from build123d import *

# Parameters (mm, degrees)
SKETCH_1_R          = 16
SKETCH_1_R_2        = 8
EXTRUDE_1_DEPTH     = 14
SKETCH_2_R          = 20
SKETCH_2_R_2        = 10
CUT_EXTRUDE_1_DEPTH = 12
EXTRUDE_START       = -5
SKETCH_4_R          = 9.5
SKETCH_4_R_2        = 7.5
EXTRUDE_2_DEPTH     = 4
EXTRUDE_START_2     = 17
SKETCH_6_R          = 16
SKETCH_6_R_2        = 14
EXTRUDE_3_DEPTH     = 17
EXTRUDE_START_3     = 3
SKETCH_7_R          = 21
SKETCH_7_R_2        = 14
EXTRUDE_4_DEPTH     = 3
SKETCH_8_R          = 1.5
CUT_EXTRUDE_4_DEPTH = 10
SKETCH_11_W         = 15
SKETCH_11_H         = 15
CUT_EXTRUDE_5_DEPTH = 11


with BuildPart() as part:
    # 草图1 → 凸台-拉伸1 (new body)
    with BuildSketch(Plane(origin=(0, 0, 0), x_dir=(1, 0, 0), z_dir=(0, 1, 0))):
        with Locations(Location((0, 0, 0), (0, 0, 270))):
            Circle(SKETCH_1_R)
        with Locations(Location((0, 0, 0), (0, 0, 270))):
            Circle(SKETCH_1_R_2, mode=Mode.SUBTRACT)
    extrude(amount=EXTRUDE_1_DEPTH)

    # 草图2 → 切除-拉伸1 (cut)
    with BuildSketch(Plane(origin=(0, 14, 0), x_dir=(1, 0, 0), z_dir=(0, 1, 0))):
        Circle(SKETCH_2_R)
        with Locations(Location((0, 0, 0), (0, 0, 270))):
            Circle(SKETCH_2_R_2, mode=Mode.SUBTRACT)
    extrude(amount=-CUT_EXTRUDE_1_DEPTH, mode=Mode.SUBTRACT)

    # 草图4 → 凸台-拉伸2 (add)
    with BuildSketch(Plane.XZ.offset(EXTRUDE_START)):
        Circle(SKETCH_4_R)
        with Locations(Location((0, 0, 0), (0, 0, 270))):
            Circle(SKETCH_4_R_2, mode=Mode.SUBTRACT)
    extrude(amount=-EXTRUDE_2_DEPTH)

    # 草图6 → 凸台-拉伸3 (add)
    with BuildSketch(Plane.XZ.offset(EXTRUDE_START_2)):
        with Locations(Location((0, 0, 0), (0, 0, 270))):
            Circle(SKETCH_6_R)
        with Locations(Location((0, 0, 0), (0, 0, 270))):
            Circle(SKETCH_6_R_2, mode=Mode.SUBTRACT)
    extrude(amount=-EXTRUDE_3_DEPTH)

    # 草图7 → 凸台-拉伸4 (add)
    with BuildSketch(Plane.XZ.offset(17).offset(EXTRUDE_START_3)):
        with Locations(Location((0, 0, 0), (0, 0, 270))):
            Circle(SKETCH_7_R)
        with Locations(Location((0, 0, 0), (0, 0, 270))):
            Circle(SKETCH_7_R_2, mode=Mode.SUBTRACT)
    extrude(amount=-EXTRUDE_4_DEPTH)

    # 草图8 → 切除-拉伸4 (cut)
    with BuildSketch(Plane(origin=(0, -17, 0), x_dir=(1, 0, 0), z_dir=(0, 1, 0))):
        with Locations(Location((18.5, 0, 0), (0, 0, 270))):
            Circle(SKETCH_8_R)
        with Locations(Location((-9.25, -16.02146997, 0), (0, 0, 270))):
            Circle(SKETCH_8_R)
        with Locations(Location((-9.25, 16.02146997, 0), (0, 0, 270))):
            Circle(SKETCH_8_R)
    extrude(amount=-CUT_EXTRUDE_4_DEPTH, mode=Mode.SUBTRACT)

    # 草图11 → 切除-拉伸5 (cut, symmetric)
    with BuildSketch(Plane.XY):
        with Locations((-8.5, -8.5)):
            Rectangle(SKETCH_11_W, SKETCH_11_H)
    cut_extrude_5 = extrude(amount=CUT_EXTRUDE_5_DEPTH, both=True, mode=Mode.SUBTRACT)

    # 镜向1: 切除-拉伸5 across plane
    add(cut_extrude_5.mirror(Plane(origin=(0, 0, 0), x_dir=(0, 0, 1), z_dir=(1, 0, 0))), mode=Mode.SUBTRACT)


solid = part.part
Input: part model. Units: mm. Frame: model coordinates. A direction names the side the tool comes from. Coordinates: 2 decimals unless noted, no trailing zeros. Write each loop counter-clockwise with the first axis right and the second up, starting at its lowest first coordinate (ties: lowest second). Pieces come first, ordered by that corner, then holes. Notation, with made-up numbers: M 55,85 L 109,85 A20 cw 109,106 Z; hole C -39,-4.5 d11. An arc over 180 degrees is marked long. Answer as a JSON object with one key per item and string values. Group by question number.
(1) Set-up query: faces 1 (the face through (-9.76, 8.08, -2.17)), 2 (the face through (-10, -8, 11)), 3 (the face through (6.31, -18.52, -20.03)), 4 (the face through (-6, 0, 6)). Return all of +Z, -Z, +X, -X, +Y, -Y with unobstructed straight access to the full face (end or side cutting, diameter ignored); none if empty.
(2) Ray query, line 1 along X through (y, z) = (-18, 0); line 2 along Y through (x, z) = (13.5, -4.5); line 3 along X through (y, z) = (6.8, 0). Return the intervals inside material, ascending. Write a range as [from, to].
(3) Mould query, pull axis Y, two halves, no side actions, for faces 5 (the face through (10, -8, 11)), 6 (the face through (0.33, 6.972, 7.493)), 7 (the face through (-15.5, -17, -4.6)). Classes: pulls with the +Y half, pulls with the -Y half, needs draft (parallel to the pull), parting line crosses it, or undercut.
(4) Section B-B on x = -9.25. Give the number of separate pieces and of enclosed holes in the cut face, plus the area to 3 significant figures.
(5) Contact query for flat-ended pins moving along their axis: P1, Ø0.9, axis at x = 10.5, y = -10.5, coming from the +Z side; P2, Ø8, axis at x = -4.5, y = 0, coming from the -Z side; P3, Ø8, axis at x = 3, z = -2.5, coming from the -Y side; P4, Ø9.5, axis at x = 0, z = 0, coming from the -Y side. Output: stop coordinate, or through.
(6) Section A-A on x = 0. Output: boundary loops of the cut face in (y, z), plus the area to 3 significant figures.
(7) Section D-D on z = -12.5. Output: boundary loops of the cut face in (x, y), plus the area to 3 significant figures.
(8) Section C-C on y = 8. Output: boundary loops of the cut face in (x, z).
Result set:
{
 "1": {"face 1": "+Y", "face 2": "+X, -X", "face 3": "+Y, -Y", "face 4": "-Y"},
 "2": {"line 1": "x = [-21, -14], [14, 17], [20, 21]", "line 2": "y = [-20, -16], [-1, 2]", "line 3": "x = [-10, -7.5], [7.5, 10]"},
 "3": {"face 5": "undercut", "face 6": "needs draft", "face 7": "pulls with the +Y half"},
 "4": {"separate pieces": "3", "enclosed holes": "0", "area": "247 mm2"},
 "5": {"P1": "stops at z = 12.45", "P2": "stops at z = -15.99", "P3": "stops at y = 5", "P4": "passes through"},
 "6": {"outline": "M -20,-21 L -17,-21 L -17,-16 L 2,-16 L 2,-10 L 14,-10 L 14,-8 L 9,-8 L 9,-7.5 L 5,-7.5 L 5,-8 L 0,-8 L 0,-14 L -20,-14 Z; M -20,14 L 0,14 L 0,8 L 5,8 L 5,7.5 L 9,7.5 L 9,8 L 14,8 L 14,10 L 2,10 L 2,16 L -17,16 L -17,21 L -20,21 Z", "area": "194 mm2"},
 "7": {"outline": "M -16.87,-20 L -6.3,-20 L -6.3,0 L 6.3,0 L 6.3,-20 L 16.87,-20 L 16.87,-17 L 9.99,-17 L 9.99,2 L -9.99,2 L -9.99,-17 L -16.87,-17 Z", "area": "229 mm2"},
 "8": {"outline": "C 0,0 d20; hole C 0,0 d15"}
}
